```python
from build123d import *
from OCP.BRepFilletAPI import BRepFilletAPI_MakeChamfer

# Parameters (mm, degrees)
RESSALTO_EXTRUS_O1_DEPTH = 30
CORTE_EXTRUS_O1_REACH    = 61.169
ESBO_O2_R                = 3.25
CORTE_EXTRUS_O3_START    = 8.755336939
CORTE_EXTRUS_O3_DEPTH    = 4
CORTE_EXTRUS_O2_REACH    = 71.263
ESBO_O3_R                = 2.375
ESBO_O3_3_R              = 2.375
CORTE_EXTRUS_O4_DEPTH    = 4
ESBO_O4_W                = 6
ESBO_O4_H                = 6
ESBO_O4_W_2              = 3
RESSALTO_EXTRUS_O2_DEPTH = 1
ESBO_O5_R                = 6.5
CORTE_EXTRUS_O5_DEPTH    = 55.781368683
CHANFRO1_SIZE            = 1
ESBO_O6_W                = 10
ESBO_O6_H                = 6
RESSALTO_EXTRUS_O3_DEPTH = 1
CHANFRO2_SIZE            = 0.5
CHANFRO2_SIZE_2          = 1


# Read off the part's stored shape, not the designer's step: Corte-extrusão3
with BuildPart() as part:
    # Esboço1 → Ressalto-extrusão1 (new body)
    with BuildSketch(Plane(origin=(0, 0, 0), x_dir=(0, 0, -1), z_dir=(1, 0, 0))):
        Polygon((1.243161309, 2.755336939), (41.243161309, 2.755336939), (41.243161309, 12.755336939), (-18.756838691, 12.755336939), (-18.756838691, -9.981327227), (-11.493502857, -17.244663061), (1.243161309, -17.244663061), align=None)
    extrude(amount=RESSALTO_EXTRUS_O1_DEPTH)

    # Esboço2 → Corte-extrusão1 (cut, up to next)
    with BuildSketch(Plane(origin=(0, 12.755336939, 0), x_dir=(1, 0, 0), z_dir=(0, 1, 0)), mode=Mode.PRIVATE) as corte_extrus_o1_sk1:
        with BuildLine():
            Line((5.125, 32.834447928), (5.125, 11.243161309))
            ThreePointArc((5.125, 11.243161309), (7.5, 8.868161309), (9.875, 11.243161309))
            Line((9.875, 11.243161309), (9.875, 32.834447928))
            ThreePointArc((9.875, 32.834447928), (7.5, 35.209447928), (5.125, 32.834447928))
        make_face()
    corte_extrus_o1_tool1 = extrude(corte_extrus_o1_sk1.sketch, amount=-CORTE_EXTRUS_O1_REACH, mode=Mode.PRIVATE) & part.part
    # Esboço2 → Corte-extrusão1 (cut, up to next)
    with BuildSketch(Plane(origin=(0, 12.755336939, 0), x_dir=(1, 0, 0), z_dir=(0, 1, 0)), mode=Mode.PRIVATE) as corte_extrus_o1_sk2:
        with BuildLine():
            Line((20.125, 32.834447928), (20.125, 11.243161309))
            ThreePointArc((20.125, 11.243161309), (22.5, 8.868161309), (24.875, 11.243161309))
            Line((24.875, 11.243161309), (24.875, 32.834447928))
            ThreePointArc((24.875, 32.834447928), (22.5, 35.209447928), (20.125, 32.834447928))
        make_face()
    corte_extrus_o1_tool2 = extrude(corte_extrus_o1_sk2.sketch, amount=-CORTE_EXTRUS_O1_REACH, mode=Mode.PRIVATE) & part.part
    # Esboço2 → Corte-extrusão1 (cut, up to next)
    with BuildSketch(Plane(origin=(0, 12.755336939, 0), x_dir=(1, 0, 0), z_dir=(0, 1, 0)), mode=Mode.PRIVATE) as corte_extrus_o1_sk3:
        with Locations(Location((7.5, -7.256838691, 0), (0, 0, 270))):
            Circle(ESBO_O2_R)
    corte_extrus_o1_tool3 = extrude(corte_extrus_o1_sk3.sketch, amount=-CORTE_EXTRUS_O1_REACH, mode=Mode.PRIVATE) & part.part
    # Esboço2 → Corte-extrusão1 (cut, up to next)
    with BuildSketch(Plane(origin=(0, 12.755336939, 0), x_dir=(1, 0, 0), z_dir=(0, 1, 0)), mode=Mode.PRIVATE) as corte_extrus_o1_sk4:
        with Locations(Location((22.5, -7.256838691, 0), (0, 0, 270))):
            Circle(ESBO_O2_R)
    corte_extrus_o1_tool4 = extrude(corte_extrus_o1_sk4.sketch, amount=-CORTE_EXTRUS_O1_REACH, mode=Mode.PRIVATE) & part.part
    add(corte_extrus_o1_tool1.solids().sort_by_distance((7.5, 12.755337, -22.038805))[0], mode=Mode.SUBTRACT)
    add(corte_extrus_o1_tool2.solids().sort_by_distance((22.5, 12.755337, -22.038805))[0], mode=Mode.SUBTRACT)
    add(corte_extrus_o1_tool3.solids().sort_by_distance((7.5, 12.755337, 7.256839))[0], mode=Mode.SUBTRACT)
    add(corte_extrus_o1_tool4.solids().sort_by_distance((22.5, 12.755337, 7.256839))[0], mode=Mode.SUBTRACT)

    # Corte-extrusão3 outline → Corte-extrusão3 (cut)
    # profile 1 of 2: a face of its own
    with BuildSketch(Plane(origin=(0, 0, 0), x_dir=(1, 0, 0), z_dir=(0, 1, 0)).offset(CORTE_EXTRUS_O3_START)):
        with BuildLine():
            ThreePointArc((2.75, 11.243161309), (7.5, 6.493161309), (12.25, 11.243161309))
            Line((12.25, 11.243161309), (12.25, 32.834447928))
            ThreePointArc((12.25, 32.834447928), (7.5, 37.584447928), (2.75, 32.834447928))
            Line((2.75, 32.834447928), (2.75, 11.243161309))
        make_face()
        with BuildLine():
            ThreePointArc((5.125, 32.834447928), (7.5, 35.209447928), (9.875, 32.834447928))
            Line((9.875, 32.834447928), (9.875, 11.243161309))
            ThreePointArc((9.875, 11.243161309), (7.5, 8.868161309), (5.125, 11.243161309))
            Line((5.125, 11.243161309), (5.125, 32.834447928))
        make_face(mode=Mode.SUBTRACT)
    # profile 2 of 2: a face of its own
    with BuildSketch(Plane(origin=(0, 0, 0), x_dir=(1, 0, 0), z_dir=(0, 1, 0)).offset(CORTE_EXTRUS_O3_START)):
        with BuildLine():
            ThreePointArc((17.75, 11.243161309), (22.5, 6.493161309), (27.25, 11.243161309))
            Line((27.25, 11.243161309), (27.25, 32.834447928))
            ThreePointArc((27.25, 32.834447928), (22.5, 37.584447928), (17.75, 32.834447928))
            Line((17.75, 32.834447928), (17.75, 11.243161309))
        make_face()
        with BuildLine():
            Line((20.125, 11.243161309), (20.125, 32.834447928))
            ThreePointArc((20.125, 32.834447928), (22.5, 35.209447928), (24.875, 32.834447928))
            Line((24.875, 32.834447928), (24.875, 11.243161309))
            ThreePointArc((24.875, 11.243161309), (22.5, 8.868161309), (20.125, 11.243161309))
        make_face(mode=Mode.SUBTRACT)
    extrude(amount=CORTE_EXTRUS_O3_DEPTH, mode=Mode.SUBTRACT)

    # Esboço3 → Corte-extrusão2 (cut, up to next)
    with BuildSketch(Plane.XY.offset(18.756838691), mode=Mode.PRIVATE) as corte_extrus_o2_sk1:
        with Locations((15, -7.244663061)):
            Circle(ESBO_O3_R)
    corte_extrus_o2_tool1 = extrude(corte_extrus_o2_sk1.sketch, amount=-CORTE_EXTRUS_O2_REACH, mode=Mode.PRIVATE) & part.part
    add(corte_extrus_o2_tool1.solids().sort_by_distance((15, -7.244663, 18.756839))[0], mode=Mode.SUBTRACT)

    # Esboço3<3> → Corte-extrusão4 (cut)
    # profile 1 of 2: a face of its own
    with BuildSketch(Plane.XY.offset(18.756838691)):
        with BuildLine():
            Line((18.882417963, -9.981327227), (11.117582037, -9.981327227))
            ThreePointArc((11.117582037, -9.981327227), (15, -11.994663061), (18.882417963, -9.981327227))
        make_face()
    # profile 2 of 2: a face of its own
    with BuildSketch(Plane.XY.offset(18.756838691)):
        with BuildLine():
            ThreePointArc((18.882417963, -9.981327227), (19.527912617, -8.680109799), (19.75, -7.244663061))
            ThreePointArc((19.75, -7.244663061), (13.564553262, -2.716750444), (11.117582037, -9.981327227))
            Line((11.117582037, -9.981327227), (18.882417963, -9.981327227))
        make_face()
        with Locations((15, -7.244663061)):
            Circle(ESBO_O3_3_R, mode=Mode.SUBTRACT)
    extrude(amount=-CORTE_EXTRUS_O4_DEPTH, mode=Mode.SUBTRACT)

    # Esboço4 → Ressalto-extrusão2 (add)
    with BuildSketch(Plane.XZ.offset(-2.755336939)):
        with Locations((15, -11.243161309)):
            Rectangle(ESBO_O4_W, ESBO_O4_H)
        with Locations((1.5, -11.243161309)):
            Rectangle(ESBO_O4_W_2, ESBO_O4_H)
        with Locations((28.5, -11.243161309)):
            Rectangle(ESBO_O4_W_2, ESBO_O4_H)
    extrude(amount=RESSALTO_EXTRUS_O2_DEPTH)

    # Esboço5 → Corte-extrusão5 (cut, through all)
    with BuildSketch(Plane.XZ.offset(-2.755336939)):
        with Locations(Location((7.5, 7.256838691, 0), (0, 0, 40.677035539))):
            Circle(ESBO_O5_R)
        with Locations(Location((22.5, 7.256838691, 0), (0, 0, 40.677035539))):
            Circle(ESBO_O5_R)
    extrude(amount=CORTE_EXTRUS_O5_DEPTH, mode=Mode.SUBTRACT)

    # Chanfro1
    chanfro1_edges = [part.edges().sort_by_distance(p)[0] for p in [
        (27.25, 12.755336939, -22.038804619),
        (22.5, 12.755336939, -37.584447928),
        (17.75, 12.755336939, -22.038804619),
        (22.5, 12.755336939, -6.493161309),
        (15, 12.755336939, 18.756838691),
        (15, 12.755336939, -41.243161309),
        (30, 12.755336939, -11.243161309),
        (7.5, 12.755336939, 4.006838691),
        (22.5, 12.755336939, 4.006838691),
        (12.25, 12.755336939, -22.038804619),
        (7.5, 12.755336939, -37.584447928),
        (2.75, 12.755336939, -22.038804619),
        (7.5, 12.755336939, -6.493161309),
        (0, 12.755336939, -11.243161309),
    ]]
    chamfer(chanfro1_edges, length=CHANFRO1_SIZE)

    # Esboço6 → Ressalto-extrusão3 (add)
    with BuildSketch(Plane(origin=(0, 0, -1.243161309), x_dir=(-1, 0, 0), z_dir=(0, 0, -1))):
        with Locations((-25, -7.244663061)):
            Rectangle(ESBO_O6_W, ESBO_O6_H)
        with Locations((-5, -7.244663061)):
            Rectangle(ESBO_O6_W, ESBO_O6_H)
    extrude(amount=RESSALTO_EXTRUS_O3_DEPTH)

    # Chanfro2
    chanfro2_edges_1 = [part.edges().sort_by_distance(p)[0] for p in [
        (25, -4.244663061, -1.243161309),
    ]]
    chanfro2_side_1 = [part.faces().sort_by_distance(p)[0] for p in [
        (25, -4.234663061, -1.243161309),
    ]]
    chanfro2_edges_2 = [part.edges().sort_by_distance(p)[0] for p in [
        (5, -4.244663061, -1.243161309),
    ]]
    chanfro2_side_2 = [part.faces().sort_by_distance(p)[0] for p in [
        (5, -4.234663061, -1.243161309),
    ]]
    chanfro2 = BRepFilletAPI_MakeChamfer(part.part.solid().wrapped)
    for e in chanfro2_edges_1:
        chanfro2.Add(CHANFRO2_SIZE - 0.0001, CHANFRO2_SIZE_2 - 0.0001, e.wrapped, chanfro2_side_1[0].wrapped)
    for e in chanfro2_edges_2:
        chanfro2.Add(CHANFRO2_SIZE - 0.0001, CHANFRO2_SIZE_2 - 0.0001, e.wrapped, chanfro2_side_2[0].wrapped)
    add(Compound.cast(chanfro2.Shape()), mode=Mode.REPLACE)  # a hair under: the kernel refuses the full size


solid = part.part
```
Can you work these out from the model? Positions are in its coordinate system, mm. A direction names the side the tool comes from. Coordinates: 2 decimals unless noted, no trailing zeros. Order: outer loops, then holes, each group sorted by start corner. A loop starts at its lowest first (then second) coordinate and runs counter-clockwise, first axis right, second up.
1. If we section it at B-B (y = 5): Please give me the cut outline in (x, z) (3 decimals), then the cut area to 3 significant figures.
2. I'm going to push flat-ended pins straight in: pin 1 (2 mm diameter, centred on x = 21, z = -26, fed in from +Y); pin 2 (5 mm diameter, centred on x = 4, y = -8.5, fed in from -Z). Where does each tip first touch, or does it pass through?
3. I need wall thicknesses on line 1 (Z direction, x = 7.25, y = 3.5); line 2 (X direction, y = 7, z = -26) (3 decimals); line 3 (Z direction, x = 7.5, y = -8.25). Which ranges of each line are inside material? Lowest first, please.
4. If we section it at A-A (z = -32): Please give me the cut outline in (x, y) (3 decimals), then the cut area to 3 significant figures.
5. Thinking about a two-plate mould opening in Y: for faces 4 (the face through (17, -9, 14.757)), 5 (the face through (20.125, 6, -22)), 6 (the face through (21, 2.755, 4)), which applies, +Y half, -Y half, draft (parallel to the pull), parting line (faces both ways), or undercut?
6. If we section it at D-D (z = 2): Please give me the cut outline in (x, y) (3 decimals).
7. For faces 1 (the face through (22.45, 5.8, -8.87)), 2 (the face through (2.75, 10, -22)), 3 (the face through (28, 1.755, -11)), which set-ups out of +Z, -Z, +X, -X, +Y, -Y let a thin tool reach every point of the face, with its end or its side?
8. If we section it at C-C (x = 15): Please give me the cut outline in (y, z), then the cut area to 3 significant figures.
Entries:
1. outline: (0, -41.243) - (30, -41.243) - (30, 18.757) - (0, 18.757) - close; hole circle Ø6.5 at (7.5, 7.257); hole (5.125, -32.834) arc R2.375 ccw to (9.875, -32.834) - (9.875, -11.243) arc R2.375 ccw to (5.125, -11.243) - close; hole circle Ø6.5 at (22.5, 7.257); hole (20.125, -32.834) arc R2.375 ccw to (24.875, -32.834) - (24.875, -11.243) arc R2.375 ccw to (20.125, -11.243) - close
1. area: 1,490 mm2
2. pin 1: stops at y = 8.76
2. pin 2: stops at z = -2.24
3. line 1: z = -41.24 to -35.2, -8.88 to 4.02, 10.5 to 18.76
3. line 2: x = 0 to 5.125, 9.875 to 20.125, 24.875 to 30
3. line 3: z = -2.24 to 0.76, 13.76 to 18.76
4. outline: (0, 2.755) - (5.125, 2.755) - (5.125, 8.755) - (2.75, 8.755) - (2.75, 11.755) - (1.75, 12.755) - (1, 12.755) - (0, 11.755) - close; (9.875, 2.755) - (20.125, 2.755) - (20.125, 8.755) - (17.75, 8.755) - (17.75, 11.755) - (16.75, 12.755) - (13.25, 12.755) - (12.25, 11.755) - (12.25, 8.755) - (9.875, 8.755) - close; (24.875, 2.755) - (30, 2.755) - (30, 11.755) - (29, 12.755) - (28.25, 12.755) - (27.25, 11.755) - (27.25, 8.755) - (24.875, 8.755) - close
4. area: 164 mm2
5. face 4: undercut
5. face 5: draft
5. face 6: -Y half
6. outline: (0, -17.245) - (3.677, -17.245) - (3.677, 2.755) - (11.323, 2.755) - (11.323, -17.245) - (18.677, -17.245) - (18.677, 2.755) - (26.323, 2.755) - (26.323, -17.245) - (30, -17.245) - (30, 11.755) - (29, 12.755) - (1, 12.755) - (0, 11.755) - close; hole circle Ø4.75 at (15, -7.245)
7. face 1: +Y, -Y
7. face 2: +Y
7. face 3: -Z, +X, -X, -Y
8. outline: (-17.24, -1.24) - (-9.62, -1.24) - (-9.62, 14.76) - (-11.99, 14.76) - (-11.99, 16.74) - (-17.24, 11.49) - close; (-4.87, -1.24) - (2.76, -1.24) - (2.76, -8.24) - (1.76, -8.24) - (1.76, -14.24) - (2.76, -14.24) - (2.76, -41.24) - (11.76, -41.24) - (12.76, -40.24) - (12.76, 17.76) - (11.76, 18.76) - (-2.49, 18.76) - (-2.49, 14.76) - (-4.87, 14.76) - close
8. area: 867 mm2
